Print and shaded views of the part. All mm, measured from the part's lowest x, y and z. Give positions to 0.01 mm unless a question says otherwise; leave off trailing zeros. Write each loop counter-clockwise with the first axis right and the second up, starting at its lowest first coordinate (ties: lowest second). Pieces come first, ordered by that corner, then holes. Notation, with made-up numbers: (73, -9.5) -> (96, -9.5) arc R28 cw to (96, 14.5) -> close; hole circle Ø4 at (-4, 20). An arc over 180 degrees is marked (long way). Put each result on its own line as item: value.
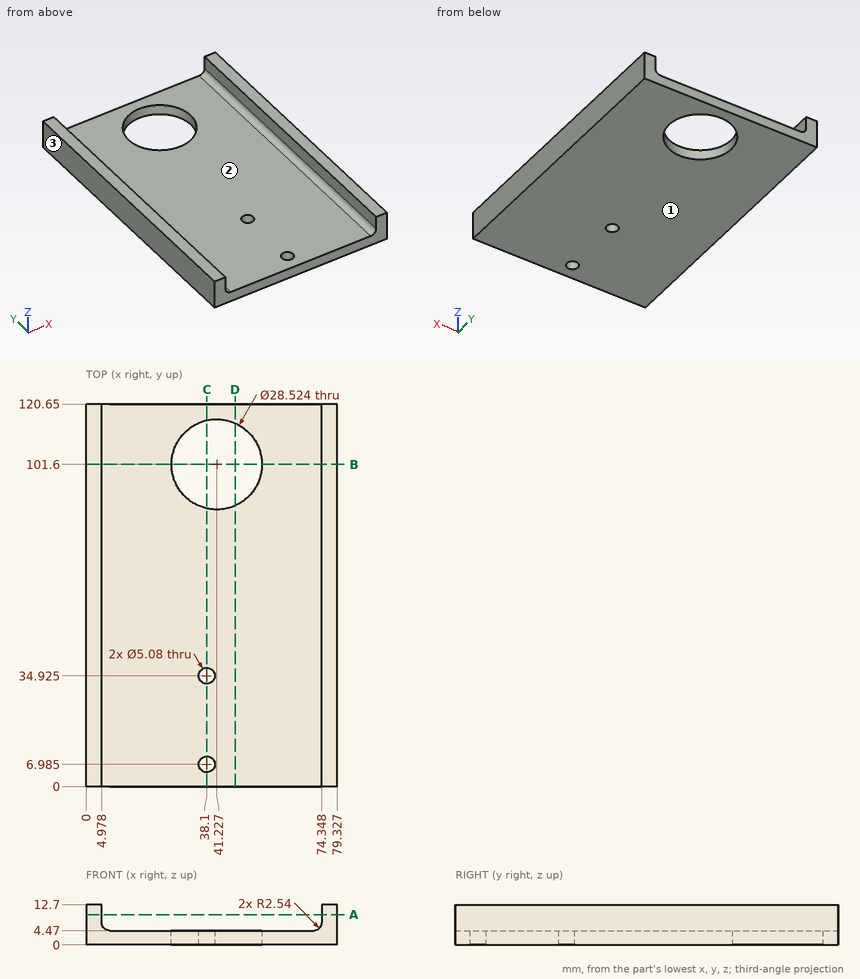
1) Slice it at B-B (y = 101.6). Write the cut outline in (x, z) (1 decimal).
Filled sheet:
outline: (0, 0) -> (27, 0) -> (27, 4.5) -> (7.5, 4.5) arc R2.5 cw to (5, 7) -> (5, 12.7) -> (0, 12.7) -> close; (55.5, 0) -> (79.3, 0) -> (79.3, 12.7) -> (74.3, 12.7) -> (74.3, 7) arc R2.5 cw to (71.8, 4.5) -> (55.5, 4.5) -> close
2) Slice it at C-C (x = 38.1). Give the number of separate pieces and of enclosed holes in the cut face.
Filled sheet:
separate pieces: 4
enclosed holes: 0
3) Pin check, flat tips, straight feed: pin 1 (4 mm diameter, centred on x = 38.1, y = 6.985, fed in from +Z); pin 2 (19.5 mm diameter, centred on x = 42, y = 61.5, fed in from +Z). Stop position of each tip, or through.
Filled sheet:
pin 1: through
pin 2: z = 4.47
4) Wall check: L1, parallel to X at y = 74, z = 11; L2, parallel to Y at x = 41, z = 3.5; L3, parallel to Z at x = 52, y = 82. Give the ranges that are in metal, low to high.
Filled sheet:
L1: 0 to 4.98, 74.35 to 79.33
L2: 0 to 87.34, 115.86 to 120.65
L3: 0 to 4.47
5) Slice it at D-D (x = 47). Write the cut outline in (y, z), plus the area to 3 significant figures.
Filled sheet:
outline: (0, 0) -> (88.56, 0) -> (88.56, 4.47) -> (0, 4.47) -> close; (114.64, 0) -> (120.65, 0) -> (120.65, 4.47) -> (114.64, 4.47) -> close
area: 423 mm2
6) Pull direction X, two halves, no side cores. Call the marked faces 1, 2 and 3: released by +X, released by -X, zero draft, split by the parting line, or undercut.
Filled sheet:
face 1: zero draft
face 2: undercut
face 3: released by -X
7) Slice it at A-A (z = 9.5). Write the cut outline in (x, y).
Filled sheet:
outline: (0, 0) -> (4.98, 0) -> (4.98, 120.65) -> (0, 120.65) -> close; (74.35, 0) -> (79.33, 0) -> (79.33, 120.65) -> (74.35, 120.65) -> close
